Check sheet for the modelled part. Datum: model origin and axes. Units: mm. A direction names the side the tool comes from. Coordinates: 2 decimals unless noted, no trailing zeros. Order: outer loops, then holes, each group sorted by start corner. A loop starts at its lowest first (then second) coordinate and runs counter-clockwise, first axis right, second up. Notation, with made-up numbers: (82.25, 14) -> (117.25, 14) arc R28 ccw to (117.25, 49) -> close; hole circle Ø7 at (-9, 24). An arc over 180 degrees is marked (long way). Put each result on its own line as item: value. Start each with the question number.
```python
from build123d import *

# Parameters (mm, degrees)
SKETCH2_R           = 2.413
SKETCH2_W           = 31.75
SKETCH2_H           = 52.3875
BOSS_EXTRUDE1_DEPTH = 9.525
FILLET1_R           = 6.35
CUT_EXTRUDE1_REACH  = 78.018
SKETCH3_R           = 2.413
CUT_EXTRUDE2_REACH  = 78.018
SKETCH4_R           = 2.413


with BuildPart() as part:
    # Sketch2 → Boss-Extrude1 (new body)
    with BuildSketch(Plane.XY):
        Polygon((-22.225, -26.19375), (-22.225, -6.35), (-38.1, -6.35), (-38.1, 6.35), (-22.225, 6.35), (-22.225, 26.19375), (-38.1, 26.19375), (-38.1, 32.54375), (38.1, 32.54375), (38.1, 26.19375), (22.225, 26.19375), (22.225, 6.35), (38.1, 6.35), (38.1, -6.35), (22.225, -6.35), (22.225, -26.19375), (38.1, -26.19375), (38.1, -32.54375), (-38.1, -32.54375), (-38.1, -26.19375), align=None)
        with Locations(Location((-31.75, 0, 0), (0, 0, 180))):
            Circle(SKETCH2_R, mode=Mode.SUBTRACT)
        with Locations(Location((31.75, 0, 0), (0, 0, 180))):
            Circle(SKETCH2_R, mode=Mode.SUBTRACT)
        Rectangle(SKETCH2_W, SKETCH2_H, mode=Mode.SUBTRACT)
    extrude(amount=BOSS_EXTRUDE1_DEPTH)

    # Fillet1
    fillet1_edges = [part.edges().sort_by_distance(p)[0] for p in [
        (-15.875, 26.19375, 4.7625),
        (-15.875, -26.19375, 4.7625),
        (15.875, -26.19375, 4.7625),
        (15.875, 26.19375, 4.7625),
    ]]
    fillet(fillet1_edges, radius=FILLET1_R)

    # Sketch3 → Cut-Extrude1 (cut, up to next)
    with BuildSketch(Plane(origin=(0, 32.54375, 0), x_dir=(1, 0, 0), z_dir=(0, 1, 0)), mode=Mode.PRIVATE) as cut_extrude1_sk1:
        with Locations(Location((-31.75, -4.7625, 0), (0, 0, 270))):
            Circle(SKETCH3_R)
    cut_extrude1_tool1 = extrude(cut_extrude1_sk1.sketch, amount=-CUT_EXTRUDE1_REACH, mode=Mode.PRIVATE) & part.part
    # Sketch3 → Cut-Extrude1 (cut, up to next)
    with BuildSketch(Plane(origin=(0, 32.54375, 0), x_dir=(1, 0, 0), z_dir=(0, 1, 0)), mode=Mode.PRIVATE) as cut_extrude1_sk2:
        with Locations(Location((31.75, -4.7625, 0), (0, 0, 270))):
            Circle(SKETCH3_R)
    cut_extrude1_tool2 = extrude(cut_extrude1_sk2.sketch, amount=-CUT_EXTRUDE1_REACH, mode=Mode.PRIVATE) & part.part
    add(cut_extrude1_tool1.solids().sort_by_distance((-31.75, 32.54375, 4.7625))[0], mode=Mode.SUBTRACT)
    add(cut_extrude1_tool2.solids().sort_by_distance((31.75, 32.54375, 4.7625))[0], mode=Mode.SUBTRACT)

    # Sketch4 → Cut-Extrude2 (cut, up to next)
    with BuildSketch(Plane.XZ.offset(32.54375), mode=Mode.PRIVATE) as cut_extrude2_sk1:
        with Locations(Location((-31.75, 4.7625, 0), (0, 0, 90))):
            Circle(SKETCH4_R)
    cut_extrude2_tool1 = extrude(cut_extrude2_sk1.sketch, amount=-CUT_EXTRUDE2_REACH, mode=Mode.PRIVATE) & part.part
    # Sketch4 → Cut-Extrude2 (cut, up to next)
    with BuildSketch(Plane.XZ.offset(32.54375), mode=Mode.PRIVATE) as cut_extrude2_sk2:
        with Locations(Location((31.75, 4.7625, 0), (0, 0, 90))):
            Circle(SKETCH4_R)
    cut_extrude2_tool2 = extrude(cut_extrude2_sk2.sketch, amount=-CUT_EXTRUDE2_REACH, mode=Mode.PRIVATE) & part.part
    add(cut_extrude2_tool1.solids().sort_by_distance((-31.75, -32.54375, 4.7625))[0], mode=Mode.SUBTRACT)
    add(cut_extrude2_tool2.solids().sort_by_distance((31.75, -32.54375, 4.7625))[0], mode=Mode.SUBTRACT)


solid = part.part
```
1) Sectioned sample at B-B (z = 1.25). State how many separate pieces and enclosed holes the cut face has, plus the area to 3 significant figures.
2) Scan lines: line 1 along Y through (x, z) = (-24.5, 6); line 2 along Y through (x, z) = (-31.75, 2); line 3 along X through (y, z) = (-7, 6.75) (3 decimals). Record each from-to range of solid material in increasing order. Write a range as [from, to].
3) Sectioned sample at D-D (y = 8.5). Record the boundary of the cut face in (x, z) (3 decimals).
4) Mould release check, pull along X, two halves, no side actions. Record for faces 1 (the flat face through (15.875, 0, 5)), 2 (the flat face through (22.225, 16, 5)), 3 (the cylindrical face through (-29.394, -29.413, 4.239)), 4 (the flat face through (17, 0, 0)): +X half, -X half, draft (parallel to the pull), parting line (faces both ways), or undercut.
5) Gauge pin test, flat ends, axial feed: pin 1 (7.5 mm diameter, centred on x = -31.75, y = 0, fed in from -Z); pin 2 (1 mm diameter, centred on y = 13.5, z = 6, fed in from -X) (3 decimals); pin 3 (3 mm diameter, centred on x = 31.75, z = 4.76, fed in from +Y); pin 4 (1 mm diameter, centred on y = -25.5, z = 3.5, fed in from +X) (3 decimals). Record the tip position at first contact, or that the pin passes through.
6) Access from +Z, -Z, +X, -X, +Y, -Y to the whole of each face (thin tool, end or side, straight path). Record for faces 5 (the flat face through (-29, -26.194, 5)), 6 (the cylindrical face through (34.106, -29.413, 4.239)), 7 (the flat face through (30, -6.35, 5)), 8 (the flat face through (0, -26.194, 5)).
7) Sectioned sample at A-A (y = 0). Record the boundary of the cut face in (x, z) (3 decimals).
Entries:
1. separate pieces: 1
1. enclosed holes: 3
1. area: 2,030 mm2
2. line 1: y = [-32.54, -26.19], [-6.35, 6.35], [26.19, 32.54]
2. line 2: y = [-32.54, -26.19], [-6.35, -2.41], [2.41, 6.35], [26.19, 32.54]
2. line 3: x = [-22.225, -15.875], [15.875, 22.225]
3. outline: (-22.225, 0) -> (-15.875, 0) -> (-15.875, 9.525) -> (-22.225, 9.525) -> close; (15.875, 0) -> (22.225, 0) -> (22.225, 9.525) -> (15.875, 9.525) -> close
4. face 1: undercut
4. face 2: +X half
4. face 3: undercut
4. face 4: draft
5. pin 1: stops at z = 0
5. pin 2: stops at x = -22.225
5. pin 3: stops at y = 6.35
5. pin 4: stops at x = 22.225
6. face 5: +Z, -Z, -X
6. face 6: -Y
6. face 7: +Z, -Z, +X
6. face 8: +Z, -Z
7. outline: (-38.1, 0) -> (-34.163, 0) -> (-34.163, 9.525) -> (-38.1, 9.525) -> close; (-29.337, 0) -> (-15.875, 0) -> (-15.875, 9.525) -> (-29.337, 9.525) -> close; (15.875, 0) -> (29.337, 0) -> (29.337, 9.525) -> (15.875, 9.525) -> close; (34.163, 0) -> (38.1, 0) -> (38.1, 9.525) -> (34.163, 9.525) -> close
